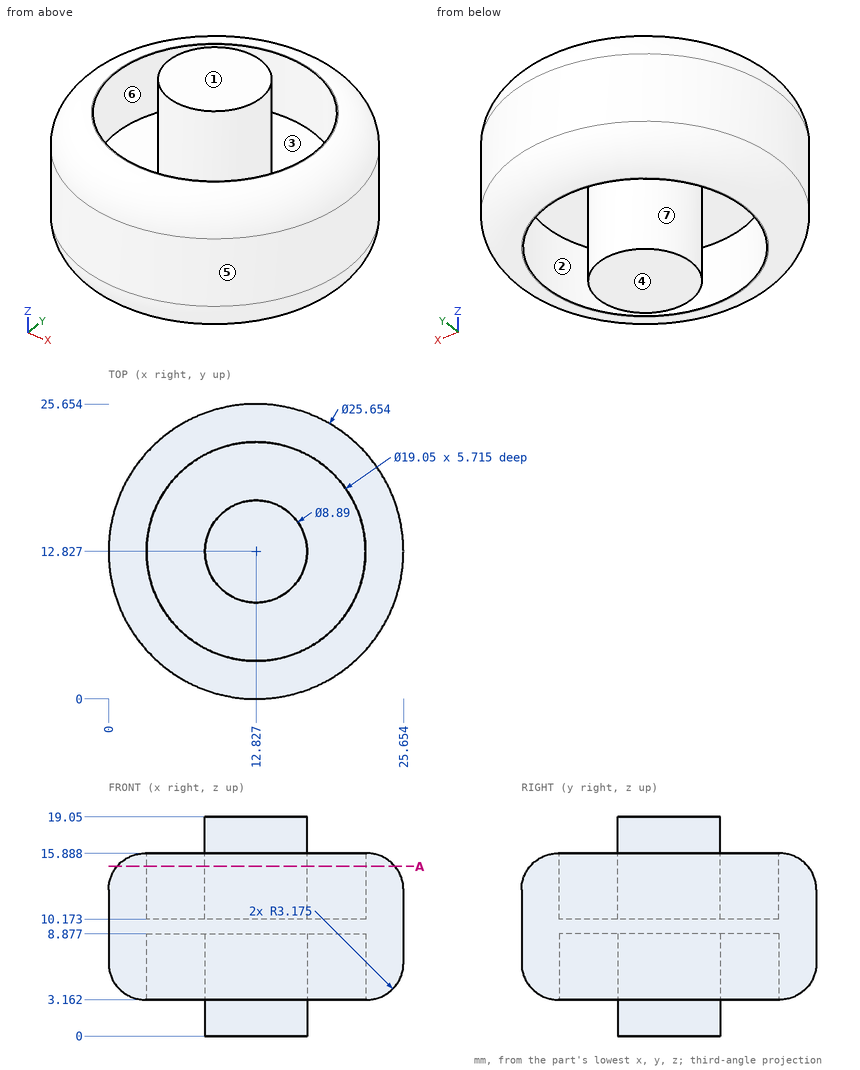
Could you check a few things on this drawing? It's one solid part, dimensions in mm from its lowest x, y, z. A direction names the side the tool comes from. Coordinates: 2 decimals unless noted, no trailing zeros.
Q1. Which directions (+Z, -Z, +X, -X, +Y, -Y) give clear straight access to the entire face, cutting with the end or side of a thin tool? Please do the marked faces 1, 2 and 3.
Results found:
face 1: +Z, +X, -X, +Y, -Y
face 2: -Z
face 3: +Z
Q2. For P1, Ø1, axis at x = 20.5, z = 15.5, coming from the +Y side; P2, Ø2, axis at x = 7, z = 16, coming from the -Y side; P3, Ø1, axis at x = 23, y = 6.5, coming from the -Z side, each with a flat end and sliding along its axis, tell me the tip position at first contact or that it passes through.
Results found:
P1: stops at y = 21.98
P2: stops at y = 2.39
P3: stops at z = 3.74
Q3. Imagine slicing it at A-A, the plane z = 14.75. Count the separate pieces of the cut face and the enclosed holes in it, plus the area to 3 significant figures.
Results found:
separate pieces: 2
enclosed holes: 1
area: 236 mm2
Q4. Please list where these lines run through material, in increasing order: L1, parallel to Y at x = 9.75, z = 10.5 (1 decimal); L2, parallel to X at y = 9.25, z = 6 (1 decimal); L3, parallel to Z at x = 16.5, y = 17.25.
Results found:
L1: y = 0.4 to 3.8, 9.6 to 16, 21.8 to 25.3
L2: x = 0.5 to 4, 10.2 to 15.5, 21.7 to 25.1
L3: z = 8.88 to 10.17
Q5. If we mould it in two halves opening along X, with no side actions, what happens to the marked faces 4, 5, 6 and 7? For each: +X half, -X half, draft (parallel to the pull), parting line (faces both ways), or undercut.
Results found:
face 4: draft
face 5: parting line
face 6: undercut
face 7: undercut
